Read the model definition and answer for the solid it produces. Units are mm, in the model's axes. Face numbers are marked on the shaded views. Coordinates: 2 decimals unless noted, no trailing zeros. Loops run counter-clockwise (first coordinate to the right, second up) from the corner with the lowest first, then second, coordinate; pieces in that order, holes last. Notation, with made-up numbers: (28, 41.25) -> (75, 41.25) arc R34 cw to (75, 75.25) -> close; hole circle Ø3 at (73.5, -37). An arc over 180 degrees is marked (long way). Answer as a JSON object with one key per item and string values. Group by question number.
Q1. The part is cut by section D-D on y = -11.5. Write down the section's boundary in (x, z).
Q2. The part is cut by section C-C on z = 20. Write down the section's boundary in (x, y), and give its area (3 significant figures).
Q3. Each of these flat-tipped pins is pushed along its axis until it touches: P1, Ø0.6, axis at x = 1.5, y = 39, coming from the +Z side; P2, Ø0.6, axis at x = 1, z = 39, coming from the -Y side. Where does it stop, or does it pass through?
Q4. The part is cut by section A-A on y = 7.5. Write down the section's boundary in (x, z), and give its area (3 significant figures).
Q5. Determine the mould class of the marked faces 1 and 2 for opening direction X: released by +X, released by -X, zero draft, split by the parting line, or undercut.
Q6. Straight lines are drawn through the part: line 1 along Y through (x, z) = (1.7, -3); line 2 along Z through (x, y) = (1.4, 11.5); line 3 along Z through (x, y) = (1.45, 26.5). For each, find the intervals that lie inside material, in ascending order. Write a range as [from, to].
Q7. The part is cut by section B-B on z = -26.5. Write down the section's boundary in (x, y).
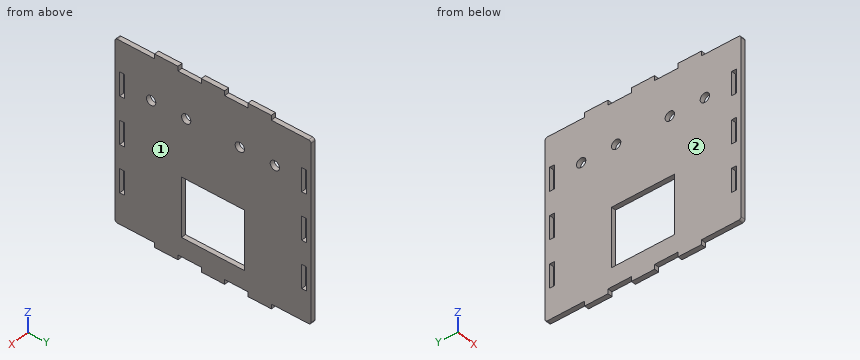
Solid Edge part; units mm, degrees
sketch "Sketch1" plane through (0, 0, 0) normal (1, 0, 0) x (0, 1, 0)
  line L0 (42, 40) -> (42, -40)
  line L1 (42, -40) -> (-42, -40)
  line L2 (-42, -40) -> (-42, 40)
  line L3 (-42, 40) -> (42, 40)
extrude "Protrusion1" add sketch "Sketch1" along normal blind 2
sketch "Sketch2" plane through (0, 0, 0) normal (1, 0, 0) x (0, 1, 0)
  line L0 (-42, 38) -> (-25, 38)
  line L1 (-25, 38) -> (-25, 40)
  line L2 (-25, 40) -> (-42, 40)
  line L3 (-42, 40) -> (-42, 38)
  line L4 (-5, 40) -> (-15, 40)
  line L5 (-15, 40) -> (-15, 38)
  line L6 (-15, 38) -> (-5, 38)
  line L7 (-5, 38) -> (-5, 40)
  line L8 (15, 40) -> (5, 40)
  line L9 (5, 40) -> (5, 38)
  line L10 (5, 38) -> (15, 38)
  line L11 (15, 38) -> (15, 40)
  line L12 (42, 40) -> (25, 40)
  line L13 (25, 40) -> (25, 38)
  line L14 (25, 38) -> (42, 38)
  line L15 (42, 38) -> (42, 40)
  line L16 (38, 25) -> (38, 15)
  line L17 (38, 15) -> (40, 15)
  line L18 (40, 15) -> (40, 25)
  line L19 (40, 25) -> (38, 25)
  line L20 (38, 5) -> (38, -5)
  line L21 (38, -5) -> (40, -5)
  line L22 (40, -5) -> (40, 5)
  line L23 (40, 5) -> (38, 5)
  line L24 (38, -15) -> (38, -25)
  line L25 (38, -25) -> (40, -25)
  line L26 (40, -25) -> (40, -15)
  line L27 (40, -15) -> (38, -15)
  line L28 (42, -38) -> (25, -38)
  line L29 (25, -38) -> (25, -40)
  line L30 (25, -40) -> (42, -40)
  line L31 (42, -40) -> (42, -38)
  line L32 (15, -38) -> (5, -38)
  line L33 (5, -38) -> (5, -40)
  line L34 (5, -40) -> (15, -40)
  line L35 (15, -40) -> (15, -38)
  line L36 (-5, -38) -> (-15, -38)
  line L37 (-15, -38) -> (-15, -40)
  line L38 (-15, -40) -> (-5, -40)
  line L39 (-5, -40) -> (-5, -38)
  line L40 (-25, -38) -> (-42, -38)
  line L41 (-42, -38) -> (-42, -40)
  line L42 (-42, -40) -> (-25, -40)
  line L43 (-25, -40) -> (-25, -38)
  line L44 (-38, -25) -> (-38, -15)
  line L45 (-38, -15) -> (-40, -15)
  line L46 (-40, -15) -> (-40, -25)
  line L47 (-40, -25) -> (-38, -25)
  line L48 (-38, 5) -> (-40, 5)
  line L49 (-40, 5) -> (-40, -5)
  line L50 (-40, -5) -> (-38, -5)
  line L51 (-38, -5) -> (-38, 5)
  line L52 (-40, 15) -> (-38, 15)
  line L53 (-38, 15) -> (-38, 25)
  line L54 (-38, 25) -> (-40, 25)
  line L55 (-40, 25) -> (-40, 15)
extrude "Cutout1" cut sketch "Sketch2" along normal blind 2
sketch "Sketch3" plane through (0, 0, 0) normal (1, 0, 0) x (0, 1, 0)
  circle A0 centre (-26.5, 20) radius 2
  circle A1 centre (-11.5, 20) radius 2
  circle A2 centre (11.5, 20) radius 2
  circle A3 centre (26.5, 20) radius 2
  line L0 (13.5, -5) -> (-13.5, -5)
  line L1 (-13.5, -5) -> (-13.5, -30)
  line L2 (-13.5, -30) -> (13.5, -30)
  line L3 (13.5, -30) -> (13.5, -5)
extrude "ExtrudedCutout_13" cut sketch "Sketch3" along normal blind 2
fillet "Round_1" radius 1 4 edges at (1, -42, -38) (1, 42, -38) (1, 42, 38) (1, -42, 38)
properties material "Acrylic, high impact grade"
Final values:
{
 "1": {"outline": "(0, -38) -> (2, -38) -> (2, -30) -> (0, -30) -> close; (0, -5) -> (2, -5) -> (2, 18) -> (0, 18) -> close; (0, 22) -> (2, 22) -> (2, 38) -> (0, 38) -> close"},
 "2": {"outline": "(0, -42) -> (2, -42) -> (2, -40) -> (0, -40) -> close; (0, -38) -> (2, -38) -> (2, -28.5) -> (0, -28.5) -> close; (0, -24.5) -> (2, -24.5) -> (2, -13.5) -> (0, -13.5) -> close; (0, -9.5) -> (2, -9.5) -> (2, 9.5) -> (0, 9.5) -> close; (0, 13.5) -> (2, 13.5) -> (2, 24.5) -> (0, 24.5) -> close; (0, 28.5) -> (2, 28.5) -> (2, 38) -> (0, 38) -> close; (0, 40) -> (2, 40) -> (2, 42) -> (0, 42) -> close", "area": "128 mm2"},
 "3": {"P1": "stops at z = 38", "P2": "stops at y = -25"},
 "4": {"outline": "(0, -38) -> (2, -38) -> (2, -30) -> (0, -30) -> close; (0, -5) -> (2, -5) -> (2, 38) -> (0, 38) -> close", "area": "102 mm2"},
 "5": {"face 1": "released by +X", "face 2": "released by -X"},
 "6": {"line 1": "y = [-42, -40], [-38, 38], [40, 42]", "line 2": "z = [-38, -30], [-5, 18], [22, 38]", "line 3": "z = [-38, 18], [22, 38]"},
 "7": {"outline": "(0, -42) -> (2, -42) -> (2, -13.5) -> (0, -13.5) -> close; (0, 13.5) -> (2, 13.5) -> (2, 42) -> (0, 42) -> close"}
}
